```python
from build123d import *

# Parameters (mm, degrees)
SKIZZE1_W                        = 42
SKIZZE1_H                        = 30
AUFSATZ_LINEAR_AUSTRAGEN1_DEPTH  = 6
SKIZZE1_3_R                      = 8.7
SCHNITT_LINEAR_AUSTRAGEN1_DEPTH  = 6
SKIZZE1_4_R                      = 11.2
SCHNITT_LINEAR_AUSTRAGEN2_DEPTH  = 3
F_5_5_5_5_DURCHMESSER_BOHRUNG1_D = 5.5
VERRUNDUNG1_R                    = 5


with BuildPart() as part:
    # Skizze1 → Aufsatz-Linear austragen1 (new body)
    with BuildSketch(Plane(origin=(0, 0, 0), x_dir=(0, 0, -1), z_dir=(1, 0, 0))):
        Rectangle(SKIZZE1_W, SKIZZE1_H)
    extrude(amount=-AUFSATZ_LINEAR_AUSTRAGEN1_DEPTH)

    # Skizze1<3> → Schnitt-Linear austragen1 (cut)
    with BuildSketch(Plane(origin=(0, 0, 0), x_dir=(0, 0, -1), z_dir=(1, 0, 0))):
        Circle(SKIZZE1_3_R)
    extrude(amount=-SCHNITT_LINEAR_AUSTRAGEN1_DEPTH, mode=Mode.SUBTRACT)

    # Skizze1<4> → Schnitt-Linear austragen2 (cut)
    with BuildSketch(Plane(origin=(0, 0, 0), x_dir=(0, 0, -1), z_dir=(1, 0, 0))):
        Circle(SKIZZE1_4_R)
    extrude(amount=-SCHNITT_LINEAR_AUSTRAGEN2_DEPTH, mode=Mode.SUBTRACT)

    # Ø5.5 (5.5) Durchmesser Bohrung1 (through all)
    with Locations(Plane(origin=(0, 0, 0), x_dir=(0, 0, -1), z_dir=(1, 0, 0))):
        with Locations((-16, 0), (16, 0)):
            Hole(F_5_5_5_5_DURCHMESSER_BOHRUNG1_D / 2)

    # Verrundung1
    verrundung1_edges = [part.edges().sort_by_distance(p)[0] for p in [
        (-3, -15, -21),
        (-3, -15, 21),
        (-3, 15, 21),
        (-3, 15, -21),
    ]]
    fillet(verrundung1_edges, radius=VERRUNDUNG1_R)


solid = part.part
```
Here's how the part is built. I have some questions about the finished solid (model axes, mm). A direction names the side the tool comes from. Coordinates: 2 decimals unless noted, no trailing zeros. Loops run counter-clockwise (first coordinate to the right, second up) from the corner with the lowest first, then second, coordinate; pieces in that order, holes last. Notation, with made-up numbers: (61, 46) - (84, 46) arc R33 ccw to (84, 76) - close; hole circle Ø3 at (-17, 11). An arc over 180 degrees is marked (long way). Return JSON: item names as keys, results as strings. Group by question number.
Item 1: Will these pins go through, and if not, where does the flat tip stop? P1, Ø3, axis at y = 3.5, z = 5.5, coming from the -X side; P2, Ø1, axis at y = 0, z = 11.5, coming from the +X side; P3, Ø11, axis at y = -3.5, z = -2, coming from the +X side.
Item 2: If we section it at C-C on y = -8: Write out the boundary of the cut face in (x, z), and give its area (3 significant figures).
Item 3: If we section it at D-D on y = -4.75: Write out the boundary of the cut face in (x, z).
Item 4: If we section it at A-A on y = 0: Write out the boundary of the cut face in (x, z), and give its area (3 significant figures).
Item 5: On a 3-axis mill with a long thin cutter (end or side, diameter ignored), from which of +Z, -Z, +X, -X, +Y, -Y can I reach the whole of each face in a straight line? I mean faces 5 (the face through (-3, -7, -6)), 6 (the face through (-3, 15, 0)). Say none if no direction works.
Item 6: If we section it at B-B on z = -18: Write out the boundary of the cut face in (x, y), and give its area (3 significant figures).
Item 7: We'd pull the mould along Z, two halves only. Please class faces 1 (the face through (-3, -15, 0)), 2 (the face through (-3.042, 0.121, 13.253)), 3 (the face through (-1.48, 0.49, 11.19)), 4 (the face through (-3, -13, 20)): +Z half, -Z half, draft (parallel to the pull), parting line (faces both ways), or undercut.
Item 8: I need wall thicknesses on line 1 (Y direction, x = -1, z = 0); line 2 (Z direction, x = -4.3, y = -0.75); line 3 (X direction, y = 1.5, z = 9). Which ranges of each line are inside material? Lowest first, please. Write a range as from..to.
Calculated:
{
 "1": {"P1": "passes through", "P2": "stops at x = 0", "P3": "stops at x = -3"},
 "2": {"outline": "(-6, -21) - (0, -21) - (0, -7.84) - (-3, -7.84) - (-3, -3.42) - (-6, -3.42) - close; (-6, 3.42) - (-3, 3.42) - (-3, 7.84) - (0, 7.84) - (0, 21) - (-6, 21) - close", "area": "184 mm^2"},
 "3": {"outline": "(-6, -21) - (0, -21) - (0, -10.14) - (-3, -10.14) - (-3, -7.29) - (-6, -7.29) - close; (-6, 7.29) - (-3, 7.29) - (-3, 10.14) - (0, 10.14) - (0, 21) - (-6, 21) - close"},
 "4": {"outline": "(-6, -21) - (0, -21) - (0, -18.75) - (-6, -18.75) - close; (-6, -13.25) - (0, -13.25) - (0, -11.2) - (-3, -11.2) - (-3, -8.7) - (-6, -8.7) - close; (-6, 8.7) - (-3, 8.7) - (-3, 11.2) - (0, 11.2) - (0, 13.25) - (-6, 13.25) - close; (-6, 18.75) - (0, 18.75) - (0, 21) - (-6, 21) - close", "area": "66.6 mm^2"},
 "5": {"face 5": "+X", "face 6": "+Z, -Z, +X, -X, +Y"},
 "6": {"outline": "(-6, -14.58) - (0, -14.58) - (0, -1.89) - (-6, -1.89) - close; (-6, 1.89) - (0, 1.89) - (0, 14.58) - (-6, 14.58) - close", "area": "152 mm^2"},
 "7": {"face 1": "draft", "face 2": "undercut", "face 3": "undercut", "face 4": "+Z half"},
 "8": {"line 1": "y = -15..-11.2, 11.2..15", "line 2": "z = -21..-18.65, -13.35..-8.67, 8.67..13.35, 18.65..21", "line 3": "x = -6..-3"}
}
